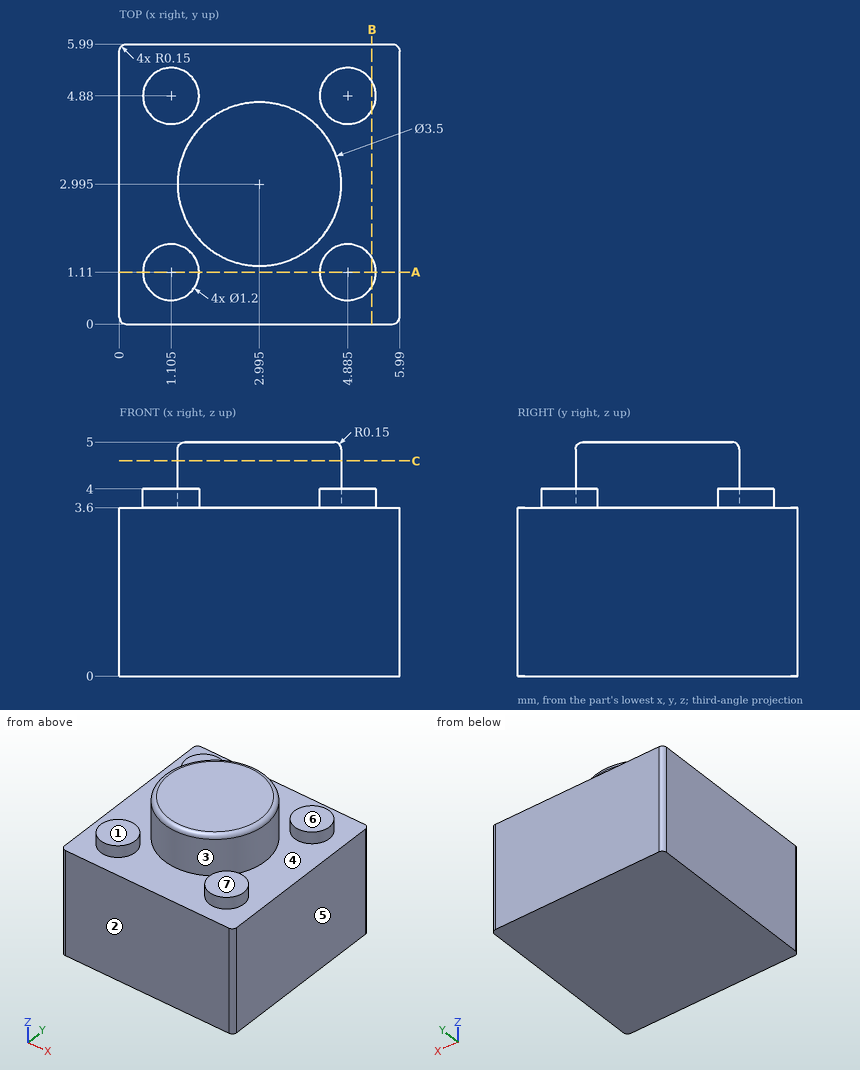
Job drawing, mm, ordinate dimensions from the low corner. One solid piece. A direction names the side the tool comes from. Round coordinates to 2 decimals unless told otherwise and drop trailing zeros. Write each loop counter-clockwise with the first axis right and the second up, starting at its lowest first coordinate (ties: lowest second). Pieces come first, ordered by that corner, then holes. Notation, with made-up numbers: (6.5, 16) -> (41.5, 16) arc R23 cw to (41.5, 51) -> close; hole circle Ø7 at (74.25, 13). An arc over 180 degrees is marked (long way). Answer as a JSON object with one key per item and string values.
(1) Probe probe 1 along Y at (x, z) = (4.4, 3.7); probe 2 along Z at (x, y) = (5.55, 5.25); probe 3 along Z at (x, y) = (4.6, 1.35). List the from-to ranges inside material, lowest first. Write a range as [from, to].
Reported:
{"probe 1": "y = [0.76, 1.46], [1.95, 4.04], [4.53, 5.23]", "probe 2": "z = [0, 3.6]", "probe 3": "z = [0, 4]"}
(2) Band-saw the part on B-B, the plane x = 5.4. List the corners of the cut face in (y, z).
Reported:
{"outline": "(0, 0) -> (5.99, 0) -> (5.99, 3.6) -> (5.19, 3.6) -> (5.19, 4) -> (4.57, 4) -> (4.57, 3.6) -> (1.42, 3.6) -> (1.42, 4) -> (0.8, 4) -> (0.8, 3.6) -> (0, 3.6) -> close"}
(3) Two-plate mould, pull along Y, no slides. Class the marked faces 1, 2, 3 and 4: +Y half, -Y half, draft (parallel to the pull), parting line (faces both ways), or undercut.
Reported:
{"face 1": "draft", "face 2": "-Y half", "face 3": "undercut", "face 4": "undercut"}
(4) Pin check, flat tips, straight feed: P1, Ø0.6, axis at x = 4.5, y = 5, coming from the +Z side; P2, Ø1, axis at y = 3.5, z = 4, coming from the +X side. Stop position of each tip, or through.
Reported:
{"P1": "stops at z = 4", "P2": "stops at x = 5.99"}
(5) Which spindle directions (+Z, -Z, +X, -X, +Y, -Y) get a long thin tool onto all of the face, cutting with end or side? Do the marked faces 5, 6 and 7. Say none if no direction does.
Reported:
{"face 5": "+Z, -Z, +X, +Y, -Y", "face 6": "+Z, +X, +Y", "face 7": "+Z, +X, -Y"}
(6) Band-saw the part on A-A, the plane y = 1.11. List the corners of the cut face in (x, z) (3 decimals), then the cut area to 3 significant figures.
Reported:
{"outline": "(0, 0) -> (5.99, 0) -> (5.99, 3.6) -> (5.485, 3.6) -> (5.485, 4) -> (4.285, 4) -> (4.285, 3.6) -> (1.705, 3.6) -> (1.705, 4) -> (0.505, 4) -> (0.505, 3.6) -> (0, 3.6) -> close", "area": "22.5 mm^2"}
(7) Band-saw the part on C-C, the plane z = 4.6. List the corners of the cut face in (x, y) (3 decimals).
Reported:
{"outline": "circle Ø3.5 at (2.995, 2.995)"}
